The model under review builds one solid part; all positions refer to its coordinate system, in mm. Round coordinates to 2 decimals unless told otherwise and drop trailing zeros. Loops run counter-clockwise (first coordinate to the right, second up) from the corner with the lowest first, then second, coordinate; pieces in that order, holes last. Notation, with made-up numbers: M -37.5,25.25 L -13.5,25.25 A14 ccw -13.5,45.25 Z; hole C 87,49.5 d4. An arc over 180 degrees is marked long. Answer as a JSON object with one key per item and string values. Group by question number.
Item 1: Consider section D-D (y = 0.8). State how many separate pieces and enclosed holes the cut face has, and give its area (3 significant figures).
Item 2: To check wall thickness, follow line 1 (X direction, y = 0.45, z = -4); line 2 (X direction, y = 1, z = 0); line 3 (Z direction, x = 10.5, y = 1.5). State the ranges of each line that lie inside material, in increasing order.
Item 3: Insertion check: P1, Ø5, axis at x = -28.448, z = -11.938, coming from the +Y side. The pin has a flat end and moves straight along its axis. Give the tip position at first contact, or say it passes through.
Item 4: Consider section B-B (z = 0). Give the boundary of the cut face in (x, y), and give its area (3 significant figures).
Item 5: Consider section C-C (x = -40.5). Give the boundary of the cut face in (y, z), and give its area (3 significant figures).
Item 6: Consider section A-A (x = -19.05). Give the boundary of the cut face in (y, z), and give its area (3 significant figures).
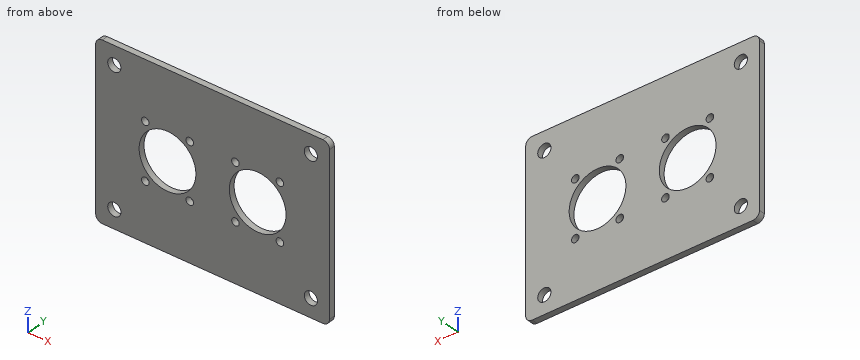
```python
from build123d import *

# Parameters (mm, degrees)
SKETCH1_R           = 12.0015
SKETCH1_R_2         = 2.794
SKETCH1_R_3         = 1.6002
BOSS_EXTRUDE1_DEPTH = 2.54


with BuildPart() as part:
    # Sketch1 → Boss-Extrude1 (new body)
    with BuildSketch(Plane(origin=(0, 0, 0), x_dir=(1, 0, 0), z_dir=(0, 1, 0))):
        with BuildLine():
            Line((-46.609, -36.703), (46.609, -36.703))
            ThreePointArc((46.609, -36.703), (48.584656347, -35.884656347), (49.403, -33.909))
            Line((49.403, -33.909), (49.403, 33.909))
            ThreePointArc((49.403, 33.909), (48.584656347, 35.884656347), (46.609, 36.703))
            Line((46.609, 36.703), (-46.609, 36.703))
            ThreePointArc((-46.609, 36.703), (-48.584656347, 35.884656347), (-49.403, 33.909))
            Line((-49.403, 33.909), (-49.403, -33.909))
            ThreePointArc((-49.403, -33.909), (-48.584656347, -35.884656347), (-46.609, -36.703))
        make_face()
        with Locations((-19.05, 0)):
            Circle(SKETCH1_R, mode=Mode.SUBTRACT)
        with Locations((19.05, 0)):
            Circle(SKETCH1_R, mode=Mode.SUBTRACT)
        with Locations((-41.529, 28.829)):
            Circle(SKETCH1_R_2, mode=Mode.SUBTRACT)
        with Locations((-28.448, -11.938)):
            Circle(SKETCH1_R_3, mode=Mode.SUBTRACT)
        with Locations((-9.652, -11.938)):
            Circle(SKETCH1_R_3, mode=Mode.SUBTRACT)
        with Locations((-9.652, 11.938)):
            Circle(SKETCH1_R_3, mode=Mode.SUBTRACT)
        with Locations((-28.448, 11.938)):
            Circle(SKETCH1_R_3, mode=Mode.SUBTRACT)
        with Locations((9.652, 11.938)):
            Circle(SKETCH1_R_3, mode=Mode.SUBTRACT)
        with Locations((28.448, 11.938)):
            Circle(SKETCH1_R_3, mode=Mode.SUBTRACT)
        with Locations((28.448, -11.938)):
            Circle(SKETCH1_R_3, mode=Mode.SUBTRACT)
        with Locations((9.652, -11.938)):
            Circle(SKETCH1_R_3, mode=Mode.SUBTRACT)
        with Locations((41.529, 28.829)):
            Circle(SKETCH1_R_2, mode=Mode.SUBTRACT)
        with Locations((41.529, -28.829)):
            Circle(SKETCH1_R_2, mode=Mode.SUBTRACT)
        with Locations((-41.529, -28.829)):
            Circle(SKETCH1_R_2, mode=Mode.SUBTRACT)
    extrude(amount=BOSS_EXTRUDE1_DEPTH)


solid = part.part
```
Geometry results:
{
 "1": {"separate pieces": "1", "enclosed holes": "14", "area": "6,180 mm^2"},
 "2": {"line 1": "x = -49.4 to -30.37, -7.73 to 7.73, 30.37 to 49.4", "line 2": "x = -49.4 to -31.05, -7.05 to 7.05, 31.05 to 49.4", "line 3": "z = -36.7 to -13.3, -10.58 to -8.42, 8.42 to 10.58, 13.3 to 36.7"},
 "3": {"P1": "stops at y = 2.54"},
 "4": {"outline": "M -49.4,0 L -31.05,0 L -31.05,2.54 L -49.4,2.54 Z; M -7.05,0 L 7.05,0 L 7.05,2.54 L -7.05,2.54 Z; M 31.05,0 L 49.4,0 L 49.4,2.54 L 31.05,2.54 Z", "area": "129 mm^2"},
 "5": {"outline": "M 0,-36.7 L 2.54,-36.7 L 2.54,-31.43 L 0,-31.43 Z; M 0,-26.23 L 2.54,-26.23 L 2.54,26.23 L 0,26.23 Z; M 0,31.43 L 2.54,31.43 L 2.54,36.7 L 0,36.7 Z", "area": "160 mm^2"},
 "6": {"outline": "M 0,-36.7 L 2.54,-36.7 L 2.54,-12 L 0,-12 Z; M 0,12 L 2.54,12 L 2.54,36.7 L 0,36.7 Z", "area": "125 mm^2"}
}
